Could you check a few things on this model? Use its own coordinates, in mm. Round coordinates to 2 decimals unless told otherwise and drop trailing zeros. Loops run counter-clockwise (first coordinate to the right, second up) from the corner with the lowest first, then second, coordinate; pieces in that order, holes last. Notation, with made-up numbers: (65.25, -33) -> (74.25, -33) arc R19 ccw to (74.25, -16) -> close; hole circle Ø1 at (63.5, 31.5). An arc over 180 degrees is marked (long way). One line per item, written item: value.
from build123d import *

# Parameters (mm, degrees)
SKETCH1_R                    = 53.721
SKETCH1_R_2                  = 50.8
TUBE_EXTRUSION_DEPTH         = 1282.7
ENGINE_BLOCK_HOLE_REACH      = 1290.312
ENGINE_BLOCK_HOLE_END_RADIUS = 50.8
SKETCH2_R                    = 1.6383
CIRPATTERN1_COUNT            = 8
SKETCH3_W                    = 5.334
SKETCH3_H                    = 203.2
FIN_SLOTS_DEPTH              = 1.27
CIRPATTERN2_COUNT            = 4


with BuildPart() as part:
    # Sketch1 → Tube Extrusion (new body)
    with BuildSketch(Plane(origin=(0, 0, 0), x_dir=(1, 0, 0), z_dir=(0, 1, 0))):
        with Locations(Location((0, 0, 0), (0, 0, 90))):
            Circle(SKETCH1_R)
        with Locations(Location((0, 0, 0), (0, 0, 90))):
            Circle(SKETCH1_R_2, mode=Mode.SUBTRACT)
    extrude(amount=TUBE_EXTRUSION_DEPTH)

    # Engine Block Hole: up to this cylinder (the profile starts outside it)
    engine_block_hole_end = Plane(origin=(0, 1066.8, 0), z_dir=(0, -1, 0)) * Cylinder(ENGINE_BLOCK_HOLE_END_RADIUS, 2683.224, mode=Mode.PRIVATE)
    # Sketch2 → Engine Block Hole (cut, up to the surface)
    with BuildSketch(Plane.XY.offset(53.721), mode=Mode.PRIVATE) as engine_block_hole_sk1:
        with Locations((0, 1066.8)):
            Circle(SKETCH2_R)
    engine_block_hole_tool1 = extrude(engine_block_hole_sk1.sketch, amount=-ENGINE_BLOCK_HOLE_REACH, mode=Mode.PRIVATE) - engine_block_hole_end
    engine_block_hole = engine_block_hole_tool1.solids().sort_by_distance((0, 1066.8, 53.721))[0]
    add(engine_block_hole, mode=Mode.SUBTRACT)

    # CirPattern1: Engine Block Hole ×8 about axis
    cirpattern1_axis = Axis((0, 1282.7, 0), (0, -1, 0))
    for i in range(1, CIRPATTERN1_COUNT):
        add(engine_block_hole.rotate(cirpattern1_axis, i * 360 / CIRPATTERN1_COUNT), mode=Mode.SUBTRACT)

    # Sketch3 → Fin Slots (cut)
    with BuildSketch(Plane.XY.offset(53.721)):
        with Locations((0, 127)):
            Rectangle(SKETCH3_W, SKETCH3_H)
    fin_slots = extrude(amount=-FIN_SLOTS_DEPTH, mode=Mode.SUBTRACT)

    # CirPattern2: Fin Slots ×4 about axis
    cirpattern2_axis = Axis((0, 0, 0), (0, 1, 0))
    for i in range(1, CIRPATTERN2_COUNT):
        add(fin_slots.rotate(cirpattern2_axis, i * 360 / CIRPATTERN2_COUNT), mode=Mode.SUBTRACT)


solid = part.part
(1) If we section it at A-A, the plane z = 15: Please give me the cut outline in (x, y), then the cut area to 3 significant figures.
Recorded:
outline: (-51.58, 0) -> (-48.53, 0) -> (-48.53, 1282.7) -> (-51.58, 1282.7) -> close; (48.53, 0) -> (51.58, 0) -> (51.58, 1282.7) -> (48.53, 1282.7) -> close
area: 7,820 mm²
(2) If I drill on L1, parallel to Z at x = -2.5, y = 1218; L2, parallel to Y at x = 51.65, z = 0; L3, parallel to Z at x = 5, y = 1221.5, over which ranges is the centre line in solid material (lowest first)?
Recorded:
L1: -53.66 to -50.74, 50.74 to 53.66
L2: 0 to 1065.16, 1068.44 to 1282.7
L3: -53.49 to -50.55, 50.55 to 53.49
(3) I'm going to push flat-ended pins straight in: pin 1 Ø4 at (y, z) = (1066.8, 0) entering from +X; pin 2 Ø3 at (y, z) = (670, -36.5) entering from -X; pin 3 Ø1 at (y, z) = (1122, -9) entering from -X; pin 4 Ø2 at (x, y) = (-14, 149) entering from -Z. Where does each tip first touch, or does it pass through?
Recorded:
pin 1: x = 53.72
pin 2: x = -40.75
pin 3: x = -53.04
pin 4: z = -52.12
(4) Thinking about a two-plate mould opening in X: for faces 1 (the face through (-15.259, 632.371, -48.454)), 2 (the face through (20.575, 632.371, -49.625)), 3 (the face through (-32, 1282.7, -40)), which applies, released by +X, released by -X, zero draft, split by the parting line, or undercut?
Recorded:
face 1: undercut
face 2: split by the parting line
face 3: zero draft
(5) If we section it at B-B, the plane y = 977: Please give me the cut outline in (x, z), then the cut area to 3 significant figures.
Recorded:
outline: circle Ø107.44 at (0, 0); hole circle Ø101.6 at (0, 0)
area: 959 mm²
